Model file for the job. Use its own axes, mm. A direction names the side the tool comes from. Round coordinates to 2 decimals unless told otherwise and drop trailing zeros. Order: outer loops, then holes, each group sorted by start corner. A loop starts at its lowest first (then second) coordinate and runs counter-clockwise, first axis right, second up. Notation, with made-up numbers: (71.5, 54) - (99.5, 54) arc R32 ccw to (99.5, 81) - close; hole circle Ø9 at (54.25, 11). An arc over 180 degrees is marked (long way). Put each result on its own line as item: value. Start each with the question number.
Item 1: Pin check, flat tips, straight feed: pin 1 Ø8 at (y, z) = (-133, -194) entering from +X; pin 2 Ø1.5 at (x, z) = (-74.5, 68) entering from -Y; pin 3 Ø2 at (x, z) = (312, 195.5) entering from +Y. Stop position of each tip, or through.
Item 2: Which spindle directions (+Z, -Z, +X, -X, +Y, -Y) get a long thin tool onto all of the face, cutting with end or side? Do faces 4 (the face through (63, 4, -70)), 5 (the face through (68.96, 169.36, 0.98)), 6 (the face through (63, 4, 70)). Say none if no direction does.
Item 3: Saw through at D-D on y = 406. List the corners of the cut face in (x, z).
Item 4: Saw through at B-B on y = -184.5. State how many separate pieces and enclosed holes the cut face has, plus the area to 3 significant figures.
Item 5: Saw through at C-C on x = 492. List the corners of the cut face in (y, z), plus the area to 3 significant figures.
Item 6: Mould opens along X. For faces 1 (the face through (182.38, -13.25, 0.98)), 2 (the face through (576.108, 181.425, 3.5)), 3 (the face through (-277, -126, 250)) say: pulls with the +X half, pulls with the -X half, needs draft (parallel to the pull), parting line crosses it, or undercut.
Item 7: Probe probe 1 along X at (y, z) = (-8, 114); probe 2 along Y at (x, z) = (0, 187); probe 3 along Y at (x, z) = (166.5, 19). List the from-to ranges inside material, lowest first.
Item 8: Saw through at A-A on z = -118. List the corners of the cut face in (x, y), plus the area to 3 significant figures.
```python
from build123d import *

# Parameters (mm, degrees)
SKETCH1_R                = 604
BOSS_EXTRUDE1_DEPTH      = 250
BOSS_EXTRUDE1_DEPTH_BACK = 250
BOSS_EXTRUDE2_DEPTH      = 70
BOSS_EXTRUDE2_DEPTH_BACK = 70
SKETCH2_R                = 13.799006552
CUT_EXTRUDE1_DEPTH       = 251
CUT_EXTRUDE1_DEPTH_BACK  = 80


with BuildPart() as part:
    # Sketch1 → Boss-Extrude1 (new body, two sides)
    with BuildSketch(Plane.XY) as boss_extrude1_sk:
        Circle(SKETCH1_R)
        with BuildLine():
            ThreePointArc((110.905261025, -283.047739926), (0, -304), (-110.905261025, -283.047739926))
            ThreePointArc((-110.905261025, -283.047739926), (-289.121180954, -93.94116629), (-256.095528158, 163.801954987))
            ThreePointArc((-256.095528158, 163.801954987), (0, 304), (256.095528158, 163.801954987))
            ThreePointArc((256.095528158, 163.801954987), (291.778203915, 85.331586883), (304, 0))
            ThreePointArc((304, 0), (251.128651643, -171.319585349), (110.905261025, -283.047739926))
        make_face(mode=Mode.SUBTRACT)
    extrude(amount=BOSS_EXTRUDE1_DEPTH)
    extrude(boss_extrude1_sk.sketch, amount=-BOSS_EXTRUDE1_DEPTH_BACK)

    # Sketch1<3> → Boss-Extrude2 (add, two sides)
    with BuildSketch(Plane.XY) as boss_extrude2_sk:
        with BuildLine():
            ThreePointArc((-256.095528158, 163.801954987), (-289.121180954, -93.94116629), (-110.905261025, -283.047739926))
            ThreePointArc((-110.905261025, -283.047739926), (0, -304), (110.905261025, -283.047739926))
            ThreePointArc((110.905261025, -283.047739926), (251.128651643, -171.319585349), (304, 0))
            ThreePointArc((304, 0), (291.778203915, 85.331586883), (256.095528158, 163.801954987))
            ThreePointArc((256.095528158, 163.801954987), (0, 304), (-256.095528158, 163.801954987))
        make_face()
        with BuildLine():
            Line((-215.721149564, -145.012778765), (-93.240227923, -46.571430252))
            Line((-93.240227923, -46.571430252), (-15.479247226, -103.068089747))
            Line((-15.479247226, -103.068089747), (-71.253846929, -249.974418035))
            add(Edge.make_bspline(
                [(-71.253846929, -249.974418035), (-117.347044344, -241.830887845), (-156.765760089, -215.769557936)],
                knots=[0, 0, 0, 1, 1, 1], degree=2))
            add(Edge.make_bspline(
                [(-215.721149564, -145.012778765), (-193.732610785, -186.3335253), (-156.765760089, -215.769557936)],
                knots=[0, 0, 0, 1, 1, 1], degree=2))
        make_face(mode=Mode.SUBTRACT)
        with BuildLine():
            Line((71.253846929, -249.974418035), (15.479247226, -103.068089747))
            Line((15.479247226, -103.068089747), (93.240227923, -46.571430252))
            Line((93.240227923, -46.571430252), (215.721149564, -145.012778765))
            add(Edge.make_bspline(
                [(215.721149564, -145.012778765), (193.732610785, -186.3335253), (156.765760089, -215.769557936)],
                knots=[0, 0, 0, 1, 1, 1], degree=2))
            add(Edge.make_bspline(
                [(71.253846929, -249.974418035), (117.347044344, -241.830887845), (156.765760089, -215.769557936)],
                knots=[0, 0, 0, 1, 1, 1], degree=2))
        make_face(mode=Mode.SUBTRACT)
        with BuildLine():
            Line((-204.576849452, 160.351591955), (-73.104877202, 74.285362947))
            Line((-73.104877202, 74.285362947), (-102.806928829, -17.128152368))
            Line((-102.806928829, -17.128152368), (-259.758448795, -9.479907899))
            add(Edge.make_bspline(
                [(-259.758448795, -9.479907899), (-266.257072669, 36.873817082), (-253.652328097, 82.416637394)],
                knots=[0, 0, 0, 1, 1, 1], degree=2))
            add(Edge.make_bspline(
                [(-204.576849452, 160.351591955), (-237.080382538, 126.670435966), (-253.652328097, 82.416637394)],
                knots=[0, 0, 0, 1, 1, 1], degree=2))
        make_face(mode=Mode.SUBTRACT)
        with BuildLine():
            Line((259.758448795, -9.479907899), (102.806928829, -17.128152368))
            Line((102.806928829, -17.128152368), (73.104877202, 74.285362947))
            Line((73.104877202, 74.285362947), (204.576849452, 160.351591955))
            add(Edge.make_bspline(
                [(204.576849452, 160.351591955), (237.080382538, 126.670435966), (253.652328097, 82.416637394)],
                knots=[0, 0, 0, 1, 1, 1], degree=2))
            add(Edge.make_bspline(
                [(259.758448795, -9.479907899), (266.257072669, 36.873817082), (253.652328097, 82.416637394)],
                knots=[0, 0, 0, 1, 1, 1], degree=2))
        make_face(mode=Mode.SUBTRACT)
        with BuildLine():
            Line((89.285703291, 244.115512743), (48.058929069, 92.48230942))
            Line((48.058929069, 92.48230942), (-48.058929069, 92.48230942))
            Line((-48.058929069, 92.48230942), (-89.285703291, 244.115512743))
            add(Edge.make_bspline(
                [(-89.285703291, 244.115512743), (-47.20887631, 264.620160097), (0, 266.705841084)],
                knots=[0, 0, 0, 1, 1, 1], degree=2))
            add(Edge.make_bspline(
                [(89.285703291, 244.115512743), (47.20887631, 264.620160097), (0, 266.705841084)],
                knots=[0, 0, 0, 1, 1, 1], degree=2))
        make_face(mode=Mode.SUBTRACT)
    extrude(amount=BOSS_EXTRUDE2_DEPTH)
    extrude(boss_extrude2_sk.sketch, amount=-BOSS_EXTRUDE2_DEPTH_BACK)

    # Sketch2 → Cut-Extrude1 (cut, two sides)
    with BuildSketch(Plane.XY) as cut_extrude1_sk:
        Circle(SKETCH2_R)
    extrude(amount=CUT_EXTRUDE1_DEPTH, mode=Mode.SUBTRACT)
    extrude(cut_extrude1_sk.sketch, amount=-CUT_EXTRUDE1_DEPTH_BACK, mode=Mode.SUBTRACT)


solid = part.part
```
Results found:
1. pin 1: stops at x = 590.06
1. pin 2: stops at y = -599.48
1. pin 3: stops at y = 517.78
2. face 4: -Z
2. face 5: +Z, -Z
2. face 6: +Z
3. outline: (-447.19, -250) - (447.19, -250) - (447.19, 250) - (-447.19, 250) - close
4. separate pieces: 3
4. enclosed holes: 0
4. area: 361,000 mm²
5. outline: (-350.36, -250) - (350.36, -250) - (350.36, 250) - (-350.36, 250) - close
5. area: 350,000 mm²
6. face 1: undercut
6. face 2: parting line crosses it
6. face 3: needs draft
7. probe 1: x = -603.95 to -303.89, 303.89 to 603.95
7. probe 2: y = -604 to -304, 304 to 604
7. probe 3: y = -580.6 to -207.58, -105.45 to -14.02, 135.43 to 580.6
8. outline: circle Ø1208 at (0, 0); hole circle Ø608 at (0, 0)
8. area: 856,000 mm²
